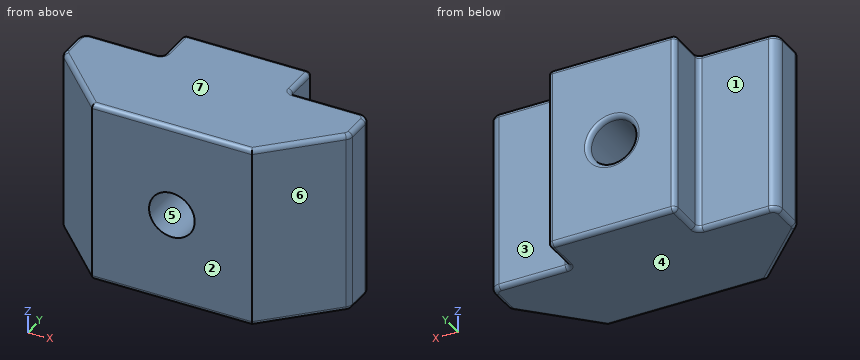
from build123d import *

# Parameters (mm, degrees)
BOSS_EXTRUDE1_DEPTH = 5
SKETCH2_R           = 1.25
CUT_EXTRUDE1_DEPTH  = 8.7
FILLET1_R           = 0.5
FILLET2_R           = 0.25


with BuildPart() as part:
    # Sketch1 → Boss-Extrude1 (new body, symmetric)
    with BuildSketch(Plane.XY):
        Polygon((-4.375, 0), (4.375, 0), (7.875, 3.5), (7.875, 5.5), (3.5, 5.5), (3.5, 7.7), (-3.5, 7.7), (-3.5, 5.5), (-7.875, 5.5), (-7.875, 3.5), align=None)
    extrude(amount=BOSS_EXTRUDE1_DEPTH, both=True)

    # Sketch2 → Cut-Extrude1 (cut, through all)
    with BuildSketch(Plane(origin=(0, 7.7, 0), x_dir=(1, 0, 0), z_dir=(0, 1, 0))):
        Circle(SKETCH2_R)
    extrude(amount=-CUT_EXTRUDE1_DEPTH, mode=Mode.SUBTRACT)

    # Fillet1
    fillet1_edges = [part.edges().sort_by_distance(p)[0] for p in [
        (7.875, 3.5, 0),
        (-7.875, 3.5, 0),
        (-7.875, 5.5, 0),
        (7.875, 5.5, 0),
    ]]
    fillet(fillet1_edges, radius=FILLET1_R)

    # Fillet2
    fillet2_edges = [part.edges().sort_by_distance(p)[0] for p in [
        (3.5, 6.6, 5),
        (-5.4375, 5.5, -5),
        (-3.5, 6.6, -5),
        (0, 7.7, -5),
        (3.5, 6.6, -5),
        (0, 7.7, 5),
        (-3.5, 6.6, 5),
        (-3.5, 5.5, 0),
        (-3.5, 7.7, 0),
        (3.5, 7.7, 0),
        (3.5, 5.5, 0),
        (-5.4375, 5.5, 5),
        (0, 0, 5),
        (-1.25, 7.7, 0),
        (6.051776695, 1.676776695, 5),
        (7.875, 4.353553391, -5),
        (7.875, 4.353553391, 5),
        (-6.051776695, 1.676776695, -5),
        (-7.875, 4.353553391, -5),
        (5.4375, 5.5, -5),
        (-7.728553391, 5.353553391, -5),
        (-7.836939766, 3.515765065, -5),
        (7.728553391, 5.353553391, -5),
        (7.836939766, 3.515765065, -5),
        (5.4375, 5.5, 5),
        (-7.875, 4.353553391, 5),
        (-6.051776695, 1.676776695, 5),
        (-7.728553391, 5.353553391, 5),
        (-7.836939766, 3.515765065, 5),
        (7.728553391, 5.353553391, 5),
        (7.836939766, 3.515765065, 5),
        (6.051776695, 1.676776695, -5),
        (0, 0, -5),
    ]]
    fillet(fillet2_edges, radius=FILLET2_R)


solid = part.part
Verification items for the finished model (mm, model axes). Face numbers are marked on the shaded views. A direction names the side the tool comes from. Coordinates: 2 decimals unless noted, no trailing zeros. Loops run counter-clockwise (first coordinate to the right, second up) from the corner with the lowest first, then second, coordinate; pieces in that order, holes last. Notation, with made-up numbers: M -29.5,51.5 L -1.5,51.5 A19 ccw -1.5,57.5 Z; hole C 1,-10.75 d1. An arc over 180 degrees is marked long. One line per item, written item: value.
1. Set-up check for the marked faces 1, 2 and 3: record each of +Z, -Z, +X, -X, +Y, -Y from which the full face is reachable in a straight line by a thin tool's end or side.
Answers follow:
face 1: +Z, -Z, -X, +Y
face 2: +Z, -Z, +X, -X, -Y
face 3: +Z, -Z, +X, +Y
2. Section check B-B on z = 0. Record the cut outline in (x, y) (3 decimals).
Answers follow:
outline: M -7.875,3.707 A0.5 ccw -7.729,3.354 L -4.375,0 L -1.25,0 L -1.25,7.45 A0.25 ccw -1.5,7.7 L -3.25,7.7 A0.25 ccw -3.5,7.45 L -3.5,5.75 A0.25 cw -3.75,5.5 L -7.375,5.5 A0.5 ccw -7.875,5 Z; M 1.25,0 L 4.375,0 L 7.729,3.354 A0.5 ccw 7.875,3.707 L 7.875,5 A0.5 ccw 7.375,5.5 L 3.75,5.5 A0.25 cw 3.5,5.75 L 3.5,7.45 A0.25 ccw 3.25,7.7 L 1.5,7.7 A0.25 ccw 1.25,7.45 Z
3. Gauge pin test, flat ends, axial feed: P1, Ø3, axis at x = -5.5, z = 0, coming from the +Y side; P2, Ø1.5, axis at y = 1.5, z = -3, coming from the +X side (3 decimals); P3, Ø1.9, axis at y = 7, z = 2, coming from the -X side. Record the tip position at first contact, or that the pin passes through.
Answers follow:
P1: y = 5.5
P2: x = 6.625
P3: x = -3.5
4. Mould release check, pull along Z, two halves, no side actions. Record for the marked faces 4, 5, 6 and 7: pulls with the +Z half, pulls with the -Z half, needs draft (parallel to the pull), parting line crosses it, or undercut.
Answers follow:
face 4: pulls with the -Z half
face 5: undercut
face 6: needs draft
face 7: pulls with the +Z half
5. Section check A-A on x = 0. Record the cut outline in (y, z).
Answers follow:
outline: M 0,-4.75 A0.25 ccw 0.25,-5 L 7.45,-5 A0.25 ccw 7.7,-4.75 L 7.7,-1.5 A0.25 ccw 7.45,-1.25 L 0,-1.25 Z; M 0,1.25 L 7.45,1.25 A0.25 ccw 7.7,1.5 L 7.7,4.75 A0.25 ccw 7.45,5 L 0.25,5 A0.25 ccw 0,4.75 Z
6. Section check C-C on z = -2.5. Record the cut outline in (x, y) (3 decimals), plus the area to 3 significant figures.
Answers follow:
outline: M -7.875,3.707 A0.5 ccw -7.729,3.354 L -4.375,0 L 4.375,0 L 7.729,3.354 A0.5 ccw 7.875,3.707 L 7.875,5 A0.5 ccw 7.375,5.5 L 3.75,5.5 A0.25 cw 3.5,5.75 L 3.5,7.45 A0.25 ccw 3.25,7.7 L -3.25,7.7 A0.25 ccw -3.5,7.45 L -3.5,5.75 A0.25 cw -3.75,5.5 L -7.375,5.5 A0.5 ccw -7.875,5 Z
area: 89.7 mm^2
7. Material ranges on line 1 along Z through (x, y) = (0, 2.75); line 2 along X through (y, z) = (5, 0) (3 decimals); line 3 along X through (y, z) = (6, 0), recorded low to high. Write a range as from..to.
Answers follow:
line 1: -5..-1.25, 1.25..5
line 2: -7.875..-1.25, 1.25..7.875
line 3: -3.5..-1.25, 1.25..3.5
